Read the model definition and answer for the solid it produces. Units are mm, in the model's axes. Coordinates: 2 decimals unless noted, no trailing zeros.
(1) Straight lines are drawn through the part: line 1 along Z through (x, y) = (-1.5, 4.5); line 2 along Z through (x, y) = (-2.4, -5.87) (3 decimals); line 3 along Y through (x, z) = (-1.3, -11). For each, find the intervals that lie inside material, in ascending order.
(2) Given pin 1 (3 mm diameter, centred on x = -1, y = -5.5, fed in from +Z); pin 2 (2.5 mm diameter, centred on y = -5.5, z = -11, fed in from +X); pin 3 (3 mm diameter, centred on x = -1, y = 2, fed in from +Z), each flat-ended and moving along its own axis, determine where each tip first touches the part or whether it passes through.
(3) The part is cut by section A-A, the plane x = 0.5. State how many separate pieces and enclosed holes the cut face has, and give its area (3 significant figures).
```python
from build123d import *

# Parameters (mm, degrees)
BOSS_EXTRUDE1_START     = -2.5
BOSS_EXTRUDE1_OUTLINE_R = 2.075
BOSS_EXTRUDE1_DEPTH     = 5
FILLET1_R               = 10
FILLET2_R               = 2
SKETCH6_R               = 2.6
CUT_EXTRUDE3_DEPTH      = 0.6
CUT_EXTRUDE4_START      = -0.6
SKETCH7_R               = 2.6
CUT_EXTRUDE4_DEPTH      = 0.6


# Read off the part's stored shape, not the designer's step: Boss-Extrude1
with BuildPart() as part:
    # Boss-Extrude1 outline → Boss-Extrude1 (new body)
    with BuildSketch(Plane(origin=(0, 0, 0), x_dir=(0, 0, -1), z_dir=(1, 0, 0)).offset(BOSS_EXTRUDE1_START)):
        with BuildLine():
            add(Edge.make_bspline(
                [(-11.466730601, 5.359735873), (-11.25264516, 5.245467231), (-10.023154699, 4.613615297), (-6.586726751, 3.178813175), (-1.892828151, 1.72609315), (2.664342093, -0.241853498), (5.954936132, -1.791511585), (8.378645161, -2.904482128), (9.714889181, -3.469566052), (9.963523485, -3.57272868)],
                knots=[0.098312483, 0.098312483, 0.098312483, 0.098312483, 0.125, 0.25, 0.5, 0.625, 0.75, 0.875, 0.903535222, 0.903535222, 0.903535222, 0.903535222], degree=3))
            ThreePointArc((-11.466730601, 5.359735873), (-17.18709042, 7.266876949), (-12.948862581, 2.977689575))
            add(Edge.make_bspline(
                [(-12.948862581, 2.977689575), (-12.654908429, 2.818079718), (-11.233080684, 2.082292793), (-8.617564406, 0.994573419), (-5.134340834, -0.202666732), (-1.7606679, -1.38003851), (1.486902599, -2.78360156), (4.761104026, -4.323813239), (7.2522862, -5.469616162), (8.677110193, -6.070847079), (8.961386544, -6.18832068)],
                knots=[0.09219974, 0.09219974, 0.09219974, 0.09219974, 0.125, 0.25, 0.375, 0.5, 0.625, 0.75, 0.875, 0.905961816, 0.905961816, 0.905961816, 0.905961816], degree=3))
            ThreePointArc((8.961386544, -6.18832068), (14.939800335, -6.979112718), (9.963523485, -3.57272868))
        make_face()
        with Locations((12.045, -5.87)):
            Circle(BOSS_EXTRUDE1_OUTLINE_R, mode=Mode.SUBTRACT)
        with Locations((-14.555, 5.629165125)):
            Circle(BOSS_EXTRUDE1_OUTLINE_R, mode=Mode.SUBTRACT)
    extrude(amount=BOSS_EXTRUDE1_DEPTH)

    # Fillet1
    fillet1_edges = [part.edges().sort_by_distance(p)[0] for p in [
        (0, -6.18832068, -8.961386544),
        (0, 5.359735873, 11.466730601),
    ]]
    fillet(fillet1_edges, radius=FILLET1_R)

    # Fillet2
    fillet2_edges = [part.edges().sort_by_distance(p)[0] for p in [
        (0, -3.57272868, -9.963523485),
        (0, 2.977689575, 12.948862581),
    ]]
    fillet(fillet2_edges, radius=FILLET2_R)

    # Sketch6 → Cut-Extrude3 (cut)
    with BuildSketch(Plane(origin=(2.5, 0, 0), x_dir=(0, 0, -1), z_dir=(1, 0, 0))):
        with Locations((-14.555, 5.629165125)):
            Circle(SKETCH6_R)
        with Locations((12.045, -5.87)):
            Circle(SKETCH6_R)
    extrude(amount=-CUT_EXTRUDE3_DEPTH, mode=Mode.SUBTRACT)

    # Sketch7 → Cut-Extrude4 (cut)
    with BuildSketch(Plane.ZY.offset(2.5).offset(CUT_EXTRUDE4_START)):
        with Locations(Location((14.555, 5.629165125, 0), (0, 0, 180))):
            Circle(SKETCH7_R)
        with Locations(Location((-12.045, -5.87, 0), (0, 0, 180))):
            Circle(SKETCH7_R)
    extrude(amount=CUT_EXTRUDE4_DEPTH, mode=Mode.SUBTRACT)


solid = part.part
```
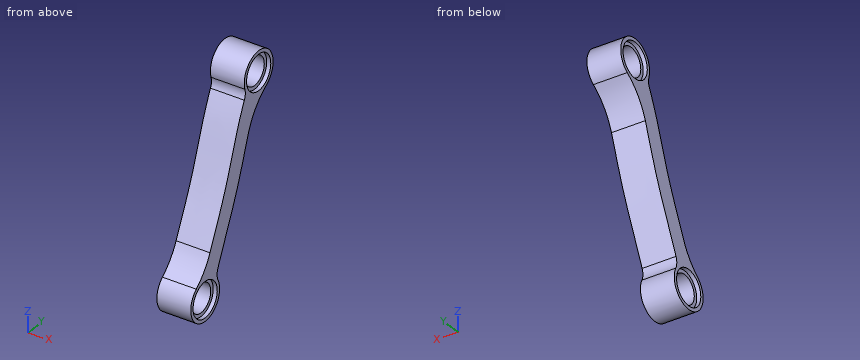
Computed:
1. line 1: z = 9.14 to 12.81, 16.3 to 17.44
1. line 2: z = -15.145 to -14.645, -9.445 to -7.639
1. line 3: y = -8.79 to -7.66, -4.08 to -2.95
2. pin 1: stops at z = -4.08
2. pin 2: stops at x = 1.9
2. pin 3: stops at z = 16.81
3. separate pieces: 1
3. enclosed holes: 2
3. area: 101 mm2
